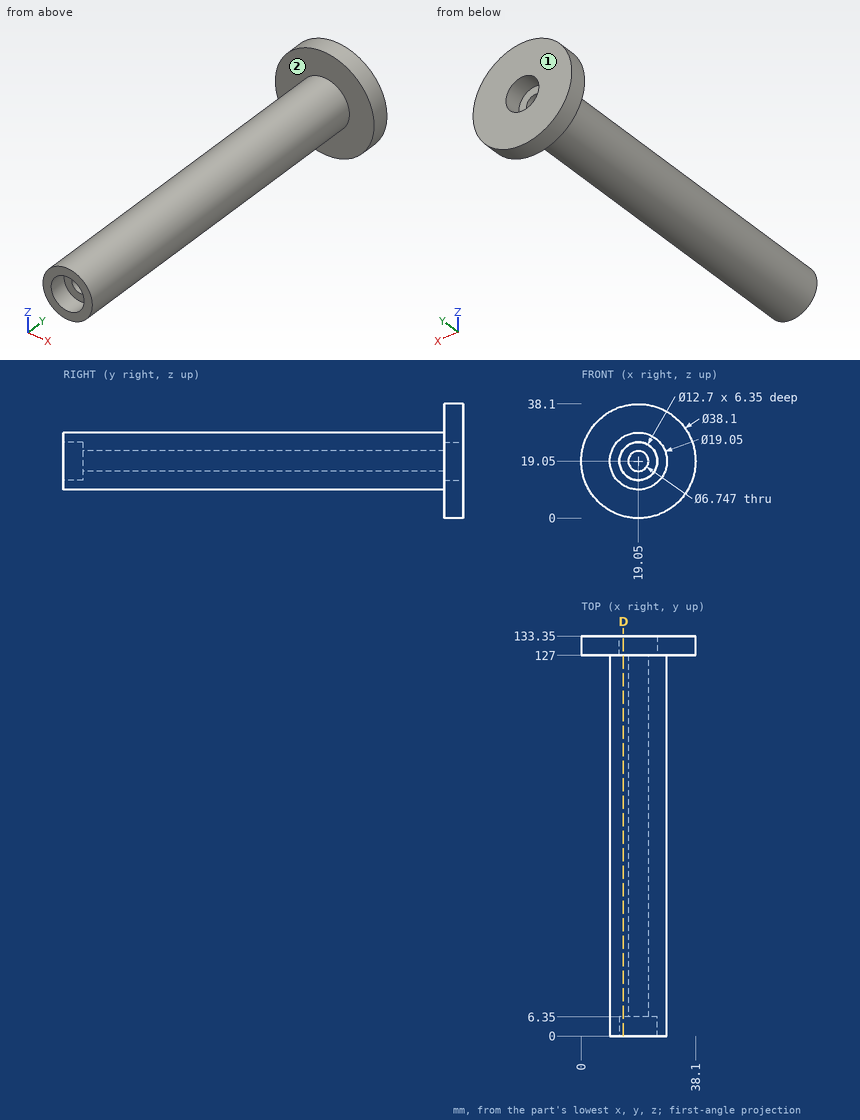
Study the drawing (mm; zero at the part's minimum x, y, z) and answer. A direction names the side the tool comes from. Coordinates: 2 decimals unless noted, no trailing zeros. Write each loop counter-clockwise with the first axis right and the second up, starting at its lowest first coordinate (ties: lowest second). Pieces come first, ordered by that corner, then holes.
Q1. Section D-D, the plane x = 14 is taken. Write down the section's boundary in (y, z).
Returned:
outline: (0, 10.97) - (127, 10.97) - (127, 0.68) - (133.35, 0.68) - (133.35, 15.2) - (127, 15.2) - (127, 22.9) - (133.35, 22.9) - (133.35, 37.42) - (127, 37.42) - (127, 27.13) - (0, 27.13) - (0, 22.9) - (6.35, 22.9) - (6.35, 15.2) - (0, 15.2) - close
Q2. Given P1, Ø3, axis at x = 10, z = 31, coming from the -Y side; P2, Ø3, axis at y = 74.5, z = 15.5, coming from the +X side; P3, Ø2, axis at y = 24.5, z = 23.5, coming from the +X side, each flat-ended and moving along its own axis, determine where each tip first touches the part or whether it passes through.
Returned:
P1: stops at y = 127
P2: stops at x = 28.35
P3: stops at x = 27.93
Q3. Find the intervals of material crossed by line 1 along Z through (x, y) = (19.05, 4.75) (3 decimals); line 2 along X through (y, z) = (129, 19); line 3 along Z through (x, y) = (19.05, 62) (1 decimal), in increasing order.
Returned:
line 1: z = 9.525 to 12.7, 25.4 to 28.575
line 2: x = 0 to 12.7, 25.4 to 38.1
line 3: z = 9.5 to 15.7, 22.4 to 28.6
Q4. Which of the six approach directions +Z, -Z, +X, -X, +Y, -Y give full straight-line access (tool end or side, diameter ignored) to the marked faces 1 and 2?
Returned:
face 1: +Z, -Z, +X, -X, +Y
face 2: -Y
